from build123d import *

# Parameters (mm, degrees)
SK_P01_STANDOFF_R           = 2.5
P01_STANDOFF_DEPTH          = 4
SK_P02_STANDOFF_R           = 2.5
P02_STANDOFF_DEPTH          = 4
SK_P03_STANDOFF_R           = 2.5
P03_STANDOFF_DEPTH          = 4
SK_P04_STANDOFF_R           = 2.5
P04_STANDOFF_DEPTH          = 4
P05_MICARRAYBOARD70MM_START = 4
SK_P05_MICARRAYBOARD70MM_R  = 35
P05_MICARRAYBOARD70MM_DEPTH = 1.6
P06_DSPANDLEDS_START        = 5.6
SK_P06_DSPANDLEDS_R         = 12
P06_DSPANDLEDS_DEPTH        = 4


with BuildPart() as part:
    # SK_P01_Standoff → P01_Standoff (new body)
    with BuildSketch(Plane(origin=(0, 0, 0), x_dir=(1, 0, 0), z_dir=(0, 1, 0))):
        with Locations(Location((21.222, -21.205, 0), (0, 0, 270))):
            Circle(SK_P01_STANDOFF_R)
    extrude(amount=P01_STANDOFF_DEPTH)



with BuildPart() as body_2:
    # SK_P02_Standoff → P02_Standoff (new body)
    with BuildSketch(Plane(origin=(0, 0, 0), x_dir=(1, 0, 0), z_dir=(0, 1, 0))):
        with Locations(Location((-21.209, -21.217, 0), (0, 0, 270))):
            Circle(SK_P02_STANDOFF_R)
    extrude(amount=P02_STANDOFF_DEPTH)


with BuildPart() as body_3:
    # SK_P03_Standoff → P03_Standoff (new body)
    with BuildSketch(Plane(origin=(0, 0, 0), x_dir=(1, 0, 0), z_dir=(0, 1, 0))):
        with Locations(Location((-21.213, 21.213, 0), (0, 0, 270))):
            Circle(SK_P03_STANDOFF_R)
    extrude(amount=P03_STANDOFF_DEPTH)


with BuildPart() as body_4:
    # SK_P04_Standoff → P04_Standoff (new body)
    with BuildSketch(Plane(origin=(0, 0, 0), x_dir=(1, 0, 0), z_dir=(0, 1, 0))):
        with Locations(Location((21.218, 21.209, 0), (0, 0, 270))):
            Circle(SK_P04_STANDOFF_R)
    extrude(amount=P04_STANDOFF_DEPTH)


with BuildPart() as part_1:
    add(part.part)

    add(body_2.part)  # P05_Micarrayboard70mm merges body 2

    add(body_3.part)  # P05_Micarrayboard70mm merges body 3

    add(body_4.part)  # P05_Micarrayboard70mm merges body 4
    # SK_P05_Micarrayboard70mm → P05_Micarrayboard70mm (add)
    with BuildSketch(Plane(origin=(0, 0, 0), x_dir=(1, 0, 0), z_dir=(0, 1, 0)).offset(P05_MICARRAYBOARD70MM_START)):
        with Locations(Location((0, 0, 0), (0, 0, 270))):
            Circle(SK_P05_MICARRAYBOARD70MM_R)
    extrude(amount=P05_MICARRAYBOARD70MM_DEPTH)

    # SK_P06_DSPandLEDs → P06_DSPandLEDs (add)
    with BuildSketch(Plane(origin=(0, 0, 0), x_dir=(1, 0, 0), z_dir=(0, 1, 0)).offset(P06_DSPANDLEDS_START)):
        with Locations(Location((0, 0, 0), (0, 0, 270))):
            Circle(SK_P06_DSPANDLEDS_R)
    extrude(amount=P06_DSPANDLEDS_DEPTH)


solid = part_1.part
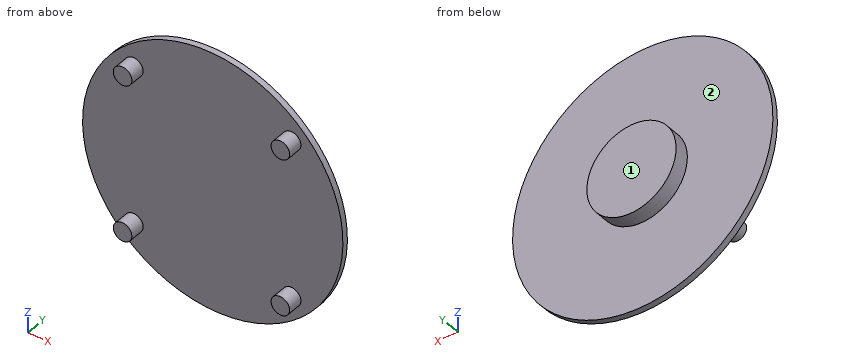
Here's how the part is built. I have some questions about the finished solid (model axes, mm). Face numbers are marked on the shaded views. A direction names the side the tool comes from. Give positions to 0.01 mm unless a question says otherwise; leave off trailing zeros. Write each loop counter-clockwise with the first axis right and the second up, starting at its lowest first coordinate (ties: lowest second). Pieces come first, ordered by that corner, then holes. Notation, with made-up numbers: (64.5, 17.25) -> (112.5, 17.25) arc R30 ccw to (112.5, 47.25) -> close; hole circle Ø4 at (24, 82). An arc over 180 degrees is marked (long way). Use one line per item in the form item = value. Start each with the question number.
1. Imagine slicing it at A-A on x = 0. List the corners of the cut face in (y, z) for me, plus the area to 3 significant figures.
2. Imagine slicing it at D-D on y = 2.25. List the corners of the cut face in (x, z) for me (3 decimals), plus the area to 3 significant figures.
3. Will these pins go through, and if not, where does the flat tip stop? pin 1 Ø8 at (x, z) = (20, -11) entering from -Y; pin 2 Ø5 at (x, z) = (18.5, 13) entering from +Y; pin 3 Ø5 at (y, z) = (4, 20) entering from -X.
4. On a 3-axis mill with a long thin cutter (end or side, diameter ignored), from which of +Z, -Z, +X, -X, +Y, -Y can I reach the whole of each face in a straight line? I mean the marked faces 1 and 2. Say none if no direction works.
5. Imagine slicing it at B-B on z = 0. List the corners of the cut face in (x, y) for me, plus the area to 3 significant figures.
6. Imagine slicing it at C-C on y = 8. List the corners of the cut face in (x, z) for me, plus the area to 3 significant figures.
7. If I drill on L1, parallel to Y at x = 10.5, z = -19.5; L2, parallel to Y at x = -3, z = 8; L3, parallel to X at y = 8, z = -3, over which ranges is the centre line in solid material (lowest first)?
Entries:
q1.outline = (4, -35) -> (5.6, -35) -> (5.6, -12) -> (9.6, -12) -> (9.6, 12) -> (5.6, 12) -> (5.6, 35) -> (4, 35) -> close
q1.area = 208 mm²
q2.outline = circle Ø5 at (-21.213, -21.213); circle Ø5 at (-21.209, 21.217); circle Ø5 at (21.218, -21.209); circle Ø5 at (21.222, 21.205)
q2.area = 78.5 mm²
q3.pin_1 = 4
q3.pin_2 = 5.6
q3.pin_3 = -30.31
q4.face_1 = +Z, -Z, +X, -X, +Y
q4.face_2 = +Y
q5.outline = (-35, 4) -> (35, 4) -> (35, 5.6) -> (12, 5.6) -> (12, 9.6) -> (-12, 9.6) -> (-12, 5.6) -> (-35, 5.6) -> close
q5.area = 208 mm²
q6.outline = circle Ø24 at (0, 0)
q6.area = 452 mm²
q7.L1 = 4 to 5.6
q7.L2 = 4 to 9.6
q7.L3 = -11.62 to 11.62
